Source: CAD feature listing. Evaluate the final solid. Frame: model axes, mm. Face numbers are marked on the shaded views. A direction names the side the tool comes from. Give positions to 0.01 mm unless a question says otherwise; leave off trailing zeros. Order: outer loops, then holes, each group sorted by start corner. A loop starts at its lowest first (then second) coordinate and runs counter-clockwise, first axis right, second up.
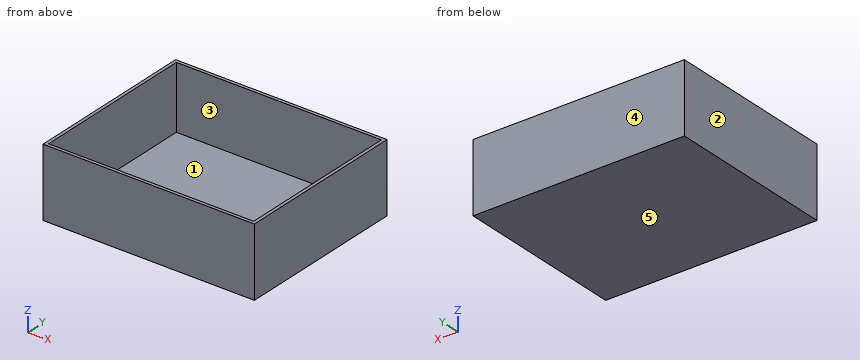
from build123d import *

# Parameters (mm, degrees)
F0_W     = 120.775796473
F0_H     = 92.5770886242
F1_DEPTH = 22
F2_DEPTH = 53.776
F3_DEPTH = 38
F5_W     = 64.999796473
F5_H     = 52.5770886242
F6_DEPTH = 20.1452


with BuildPart() as f1:
    # F0 (on Top) → F1 (new body)
    with BuildSketch(Plane.XY):
        with Locations((-0.1175701618, 19.4224845618)):
            Rectangle(F0_W, F0_H)
    extrude(amount=F1_DEPTH)

    # F2 (cut): a face of the model
    f2_faces = [f1.faces().sort_by_distance(p)[0] for p in [
        (-60.5054683983, 19.4224845618, 11),
    ]]
    extrude(f2_faces, amount=-F2_DEPTH, mode=Mode.SUBTRACT)

    # F3 (cut): a face of the model
    f3_faces = [f1.faces().sort_by_distance(p)[0] for p in [
        (26.7704298382, 65.7110288739, 11),
    ]]
    extrude(f3_faces, amount=-F3_DEPTH, mode=Mode.SUBTRACT)

    # F5 (on face) → F6 (cut)
    with BuildSketch(Plane.XY.offset(22)):
        with Locations((26.7704298382, 0.4224845618)):
            Rectangle(F5_W, F5_H)
    extrude(amount=-F6_DEPTH, mode=Mode.SUBTRACT)


solid = f1.part
(1) Access query for the marked faces 1 and 2. Directions: +Z, -Z, +X, -X, +Y, -Y. A direction counts if a zero-diameter tool reaches every point of the face in a straight line with its end or side. Return the directions, or none.
(2) Pin query (flat end, axial travel): pin 1 Ø2 at (x, y) = (49, 11.5) entering from +Z. Return the tip coordinate at first contact, or that it passes through.
(3) Draft query along Y for the marked faces 3, 4 and 5. Return one class per face: +Y half, -Y half, draft (parallel to the pull), parting line (faces both ways), or undercut.
(4) Section C-C, the plane x = -0.5. Return loops of the section in (y, z).
(5) Section B-B, the plane z = 5.5. Return loops of the section in (x, y), plus the area to 3 significant figures.
(6) Line query: line 1 along X through (y, z) = (-7.5, 12.25); line 2 along Y through (x, z) = (14.5, 6); line 3 along Z through (x, y) = (2, 5.5). Output: solid intervals per line, ascending.
(7) Section A-A, the plane y = -15.5. Return loops of the section in (x, z).
Checks:
1. face 1: +Z
1. face 2: +Z, -Z, -X, +Y, -Y
2. pin 1: stops at z = 1.85
3. face 3: undercut
3. face 4: +Y half
3. face 5: draft
4. outline: (-26.87, 0) - (27.71, 0) - (27.71, 22) - (26.71, 22) - (26.71, 1.85) - (-25.87, 1.85) - (-25.87, 22) - (-26.87, 22) - close
5. outline: (-6.73, -26.87) - (60.27, -26.87) - (60.27, 27.71) - (-6.73, 27.71) - close; hole (-5.73, -25.87) - (59.27, -25.87) - (59.27, 26.71) - (-5.73, 26.71) - close
5. area: 239 mm2
6. line 1: x = -6.73 to -5.73, 59.27 to 60.27
6. line 2: y = -26.87 to -25.87, 26.71 to 27.71
6. line 3: z = 0 to 1.85
7. outline: (-6.73, 0) - (60.27, 0) - (60.27, 22) - (59.27, 22) - (59.27, 1.85) - (-5.73, 1.85) - (-5.73, 22) - (-6.73, 22) - close
